Autodesk Inventor part; units mm, degrees
ref_plane "YZ Plane" through (0, 0, 0) normal (1, 0, 0) x (0, 1, 0)
ref_plane "XZ Plane" through (0, 0, 0) normal (0, 1, 0) x (-1, 0, 0)
ref_plane "XY Plane" through (0, 0, 0) normal (0, 0, 1) x (1, 0, 0)
sketch "Sketch1" plane through (0, 0, 0) normal (0, 1, 0) x (-1, 0, 0)
  line L0 (13.2677, 19.6408) -> (-12.1323, 19.6408)
  line L1 (-12.1323, 19.6408) -> (-12.1323, -18.4592)
  line L2 (-12.1323, -18.4592) -> (13.2677, -18.4592)
  line L3 (13.2677, -18.4592) -> (13.2677, 19.6408)
  point P0 (0, 0)
  dimension "d0" = 25.4
  dimension "d1" = 38.1
extrude "Extrusion1" add sketch "Sketch1" along normal blind 3.175
hole "Hole1" at (-9.6799, 3.175, 14.8783) direction (0, -1, 0) diameter 4.4958 depth 3.175
hole "Hole2" at (8.5446, 3.175, 14.8783) direction (0, -1, 0) diameter 4.4958 depth 3.175
hole "Hole3" at (-9.6799, 3.175, -13.6967) direction (0, -1, 0) diameter 4.4958 depth 3.175
hole "Hole4" at (8.5446, 3.175, -13.6967) direction (0, -1, 0) diameter 4.4958 depth 3.175
hole "Hole5" at (-0.5677, 3.175, -6.5466) direction (0, -1, 0) diameter 2.54 depth 3.175
hole "Hole6" at (-0.5677, 3.175, 7.7345) direction (0, -1, 0) diameter 2.54 depth 3.175
properties part number "Shield_1"
Check sheet for the modelled part. Datum: model origin and axes. Units: mm. Round coordinates to 2 decimals unless told otherwise and drop trailing zeros. Loops run counter-clockwise (first coordinate to the right, second up) from the corner with the lowest first, then second, coordinate; pieces in that order, holes last. Notation, with made-up numbers: (-36, 66) - (-11, 66) arc R31 ccw to (-11, 98) - close; hole circle Ø2 at (18.25, -29.5). An arc over 180 degrees is marked (long way). Answer as CSV lines item,"result". Start each with the question number.
Item 1: Depth check by flat-ended pin: P1, Ø5, axis at x = 8.54, z = -13.7, coming from the +Y side (3 decimals). Enter the tip coordinate at first touch or a pass-through.
Item 2: Scan lines: line 1 (X direction, y = 2.85, z = 14.5); line 2 (Z direction, x = 7.5, y = 2.7); line 3 (Z direction, x = 10, y = 2.7). Record each from-to range of solid material in increasing order. Write a range as [from, to].
Item 3: Section check D-D (z = -6). Record the boundary of the cut face in (x, y) (3 decimals).
Item 4: Release check for a two-part mould opening along X. For faces 1 (the flat face through (12.132, 2, 1)), 2 (the flat face through (0, 3.175, 1)), 3 (the cylindrical face through (8.446, 1.565, -15.942)) record: +X half, -X half, draft (parallel to the pull), parting line (faces both ways), or undercut.
Item 5: Section check B-B (x = -11). Record the boundary of the cut face in (y, z) (3 decimals).
Item 6: Section check C-C (y = 1.6). Record the boundary of the cut face in (x, z), and give its area (3 significant figures).
Item 7: Section check A-A (z = 14.5). Record the boundary of the cut face in (x, y) (3 decimals), and give its area (3 significant figures).
Report:
1,P1,"stops at y = 3.175"
2,line 1,"x = [-13.27, -11.9], [-7.46, 6.33], [10.76, 12.13]"
2,line 2,"z = [-18.46, -15.69], [-11.71, 12.89], [16.87, 19.64]"
2,line 3,"z = [-18.46, -15.41], [-11.98, 13.17], [16.59, 19.64]"
3,outline,"(-13.268, 0) - (-1.714, 0) - (-1.714, 3.175) - (-13.268, 3.175) - close; (0.579, 0) - (12.132, 0) - (12.132, 3.175) - (0.579, 3.175) - close"
4,face 1,"+X half"
4,face 2,"draft"
4,face 3,"undercut"
5,outline,"(0, -18.459) - (3.175, -18.459) - (3.175, -15.516) - (0, -15.516) - close; (0, -11.877) - (3.175, -11.877) - (3.175, 13.059) - (0, 13.059) - close; (0, 16.698) - (3.175, 16.698) - (3.175, 19.641) - (0, 19.641) - close"
6,outline,"(-13.27, -18.46) - (12.13, -18.46) - (12.13, 19.64) - (-13.27, 19.64) - close; hole circle Ø4.5 at (-9.68, -13.7); hole circle Ø4.5 at (-9.68, 14.88); hole circle Ø2.54 at (-0.57, -6.55); hole circle Ø2.54 at (-0.57, 7.73); hole circle Ø4.5 at (8.54, -13.7); hole circle Ø4.5 at (8.54, 14.88)"
6,area,"894 mm2"
7,outline,"(-13.268, 0) - (-11.896, 0) - (-11.896, 3.175) - (-13.268, 3.175) - close; (-7.464, 0) - (6.329, 0) - (6.329, 3.175) - (-7.464, 3.175) - close; (10.76, 0) - (12.132, 0) - (12.132, 3.175) - (10.76, 3.175) - close"
7,area,"52.5 mm2"
